Autodesk Inventor part; units mm, degrees
ref_plane "AS_XY" through (10.92, 0, 0) normal (1, 0, 0) x (0, 0, -1)
ref_plane "AS_YZ" through (10.92, 0, 0) normal (0, 0, -1) x (0, 1, 0)
ref_plane "AS_ZX" through (10.92, 0, 0) normal (0, 1, 0) x (1, 0, 0)
sketch "Skizze_1" plane through (0, 0, 0) normal (0, 1, 0) x (-1, 0, 0)
  line L0 (-22, 0) -> (0, 0)
  line L1 (0, 0) -> (0, -1.5705)
  line L2 (0, -1.5705) -> (-0.4295, -2)
  line L3 (-0.4295, -2) -> (-18.5, -2)
  line L4 (-18.5, -2) -> (-18.5, -1.5705)
  line L5 (-18.5, -1.5705) -> (-19.2, -1.5705)
  line L6 (-19.2, -1.5705) -> (-19.2, -4)
  line L7 (-19.2, -4) -> (-21.0872, -3.8349)
  arc A0 (-22, -2.8387) -> (-21.0872, -3.8349) centre (-21, -2.8387) ccw
  line L8 (-22, -2.8387) -> (-22, 0)
  line L9 (-22, 0) -> (0, 0)
revolve "Revolution1" add sketch "Skizze_1" angle 360 about axis through (22, 0, 0) along (1, 0, 0)
thread "Thread1"
ref_plane "AS_XY" through (10.92, 0, 0) normal (1, 0, 0) x (0, 0, -1)
ref_plane "AS_YZ" through (10.92, 0, 0) normal (0, 0, -1) x (0, 1, 0)
ref_plane "AS_ZX" through (10.92, 0, 0) normal (0, 1, 0) x (1, 0, 0)
properties part number "205-S-AS"
Work out the finished part from the listing and answer in its coordinate system (mm). A direction names the side the tool comes from. Coordinates: 2 decimals unless noted, no trailing zeros. Loops run counter-clockwise (first coordinate to the right, second up) from the corner with the lowest first, then second, coordinate; pieces in that order, holes last. Notation, with made-up numbers: M 29,-2.75 L 36,-2.75 A28 cw 36,19.25 Z; hole C 34,-8.75 d5. An arc over 180 degrees is marked long. Use CSV: the item, a comma, the result in double quotes. Start each with the question number.
(1) For faces 3 (the face through (19.2, 0, -2)), 4 (the face through (20.55, 3.79, 0.84)), determine the directions among +Z, -Z, +X, -X, +Y, -Y from which every point of the face is accessible in a straight line to the end or side of a thin tool.
(2) Given pin 1 Ø3 at (x, z) = (10, 0.5) entering from +Y; pin 2 Ø4 at (x, z) = (11.5, 2.5) entering from +Y, each flat-ended and moving along its own axis, determine where each tip first touches the part or whether it passes through.
(3) For a pull along Y with two mould halves and no side action, classify faces 1 (the face through (10, -2, 0)), 2 (the face through (22, 0, 0)) as +Y half, -Y half, draft (parallel to the pull), parting line (faces both ways), or undercut.
(4) Consider line 1 (X direction, y = 1.5, z = -2); line 2 (X direction, y = -0.5, z = 1.75); line 3 (Y direction, x = 14, z = 1.75). Determine where each line is inside the solid, lowest interval first.
(5) Find section A-A, the plane y = 0. Give the vertices of the cut face in (x, z).
(6) Find section C-C, the plane x = 10.75. Give the vertices of the cut face in (y, z), then the cut area to 3 significant figures.
Recorded:
1,face 3,"none"
1,face 4,"+X"
2,pin 1,"stops at y = 2"
2,pin 2,"stops at y = 1.94"
3,face 1,"parting line"
3,face 2,"draft"
4,line 1,"x = 19.2 to 22"
4,line 2,"x = 0.25 to 18.5, 19.2 to 22"
4,line 3,"y = -0.97 to 0.97"
5,outline,"M 0,-1.57 L 0.43,-2 L 18.5,-2 L 18.5,-1.57 L 19.2,-1.57 L 19.2,-4 L 21.09,-3.83 A1 ccw 22,-2.84 L 22,2.84 A1 ccw 21.09,3.83 L 19.2,4 L 19.2,1.57 L 18.5,1.57 L 18.5,2 L 0.43,2 L 0,1.57 Z"
6,outline,"C 0,0 d4"
6,area,"12.6 mm^2"
